Can you work these out from the drawing? Everything is in mm from the part's minimum corner. Coordinates: 2 decimals unless noted, no trailing zeros. Write each loop counter-clockwise with the first axis right and the second up, starting at its lowest first coordinate (ties: lowest second). Pieces come first, ordered by that corner, then holes.
(1) Imagine slicing it at A-A, the plane x = 96. List the corners of the cut face in (y, z) for me, plus the area to 3 significant figures.
(2) For pin 1 Ø1.5 at (y, z) = (66, 1) entering from -X; pin 2 Ø1 at (x, z) = (67.5, 2.5) entering from -Y; pin 3 Ø0.9 at (y, z) = (155, 1) entering from -X, each with a flat end and sliding along its axis, tell me the tip position at first contact or that it passes through.
(3) Please list where this line runs through material, in increasing order: probe 1 along X at (y, z) = (109.5, 1.45).
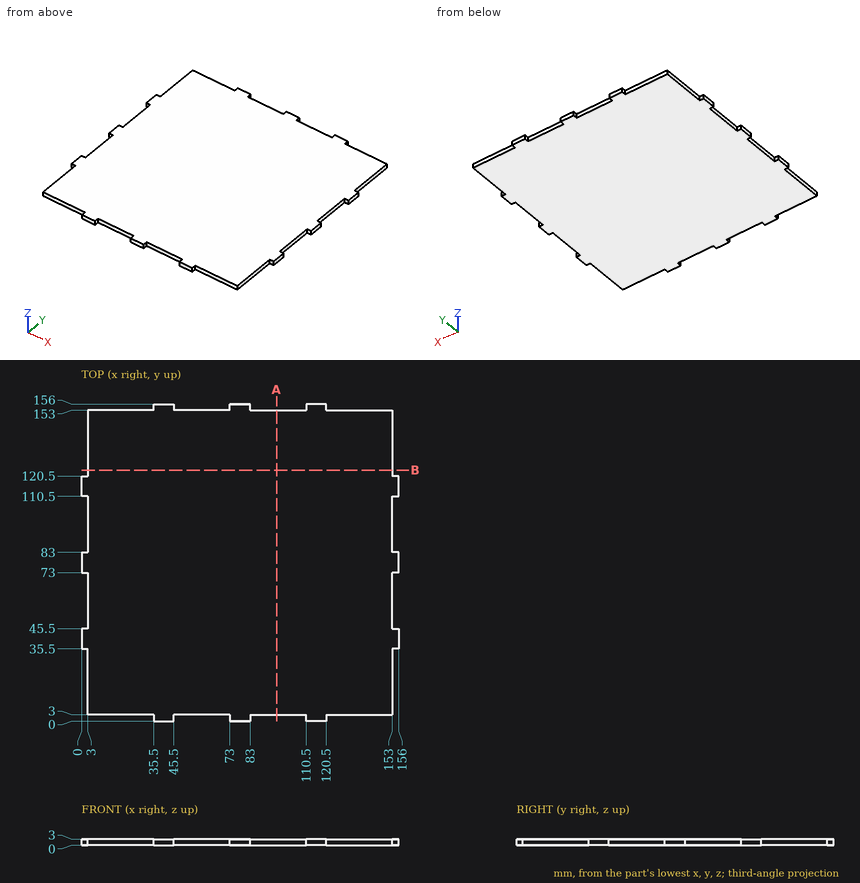
Recorded:
1. outline: (3, 0) - (153, 0) - (153, 3) - (3, 3) - close
1. area: 450 mm2
2. pin 1: stops at x = 3
2. pin 2: stops at y = 3
2. pin 3: stops at x = 35.5
3. probe 1: x = 3 to 153
